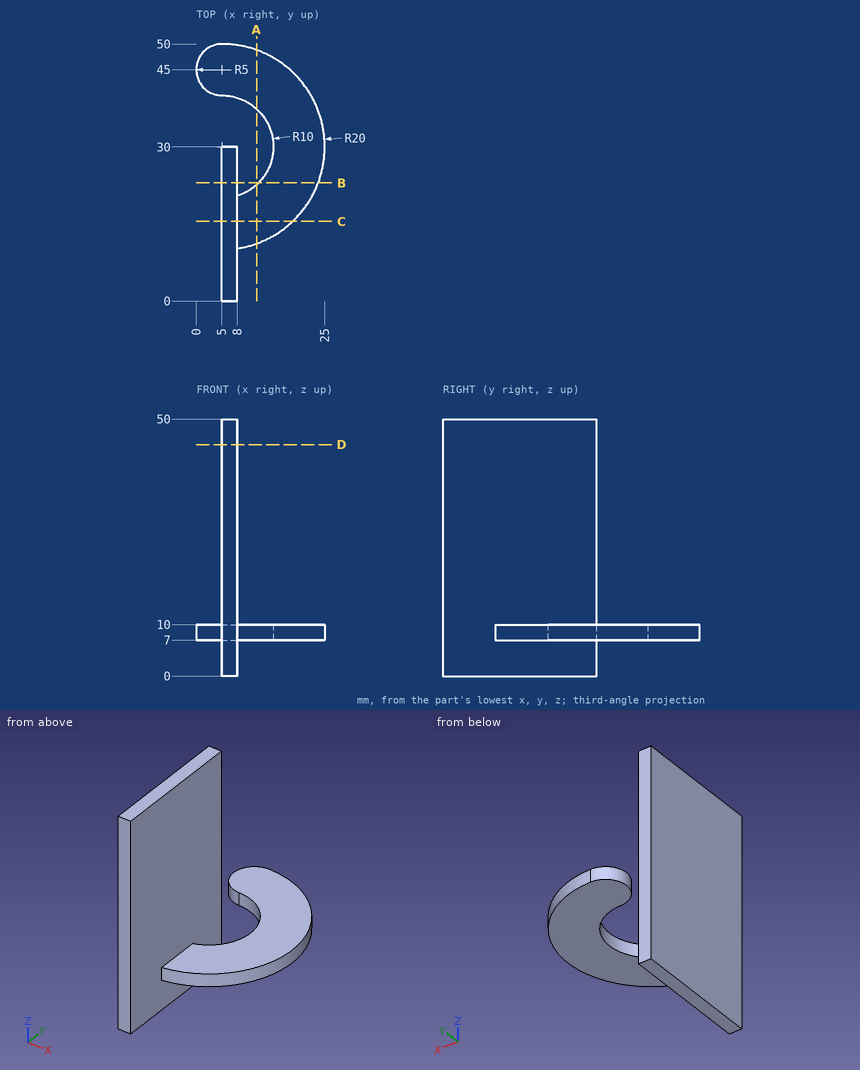
Can you work these out from the drawing? Everything is in mm from the part's minimum corner. Round coordinates to 2 decimals unless told otherwise and drop trailing zeros. Order: outer loops, then holes, each group sorted by start corner. A loop starts at its lowest first (then second) coordinate and runs counter-clockwise, first axis right, second up. Notation, with made-up numbers: M 39,46 L 75,46 A23 ccw 75,54 Z; hole C 15,-15.5 d9. An arc over 180 degrees is marked long. Answer as CSV lines item,"result".
Item 1: For pin 1 (6 mm diameter, centred on x = 13, y = 12.5, fed in from +Z); pin 2 (8 mm diameter, centred on y = 24.5, z = 31, fed in from -X); pin 3 (4 mm diameter, centred on x = 6.5, z = 22.5, fed in from +Y), each with a flat end and sliding along its axis, tell me the tip position at first contact or that it passes through.
From the geometry:
pin 1,"z = 10"
pin 2,"x = 5"
pin 3,"y = 30"
Item 2: Imagine slicing it at D-D on z = 45. List the corners of the cut face in (x, y) for me, and give its area (3 significant figures).
From the geometry:
outline,"M 5,0 L 8,0 L 8,30 L 5,30 Z"
area,"90.0 mm2"
Item 3: Imagine slicing it at B-B on y = 23. List the corners of the cut face in (x, z) for me (3 decimals), and give its area (3 significant figures).
From the geometry:
outline,"M 5,0 L 8,0 L 8,50 L 5,50 Z; M 12.141,7 L 23.735,7 L 23.735,10 L 12.141,10 Z"
area,"185 mm2"
Item 4: Imagine slicing it at C-C on y = 15.5. List the corners of the cut face in (x, z) for me.
From the geometry:
outline,"M 5,0 L 8,0 L 8,7 L 18.77,7 L 18.77,10 L 8,10 L 8,50 L 5,50 Z"
Item 5: Imagine slicing it at A-A on x = 11.75. List the corners of the cut face in (y, z) for me, and give its area (3 significant figures).
From the geometry:
outline,"M 11.17,7 L 22.62,7 L 22.62,10 L 11.17,10 Z; M 37.38,7 L 48.83,7 L 48.83,10 L 37.38,10 Z"
area,"68.7 mm2"
Item 6: Please list where these lines run through material, in increasing order: L1, parallel to Z at x = 21.5, y = 23; L2, parallel to X at y = 3, z = 23.5; L3, parallel to Y at x = 6, z = 41.5. Write a range as [from, to].
From the geometry:
L1,"[7, 10]"
L2,"[5, 8]"
L3,"[0, 30]"
